Check sheet for the modelled part. Datum: model origin and axes. Units: mm. Face numbers are marked on the shaded views. Coordinates: 2 decimals unless noted, no trailing zeros. Loops run counter-clockwise (first coordinate to the right, second up) from the corner with the lowest first, then second, coordinate; pieces in that order, holes last. Notation, with made-up numbers: M 48.25,75.5 L 101.25,75.5 A30 ccw 101.25,113.5 Z; hole C 0.5,-35.75 d4. An arc over 180 degrees is marked long. Return JSON: item names as keys, results as strings.
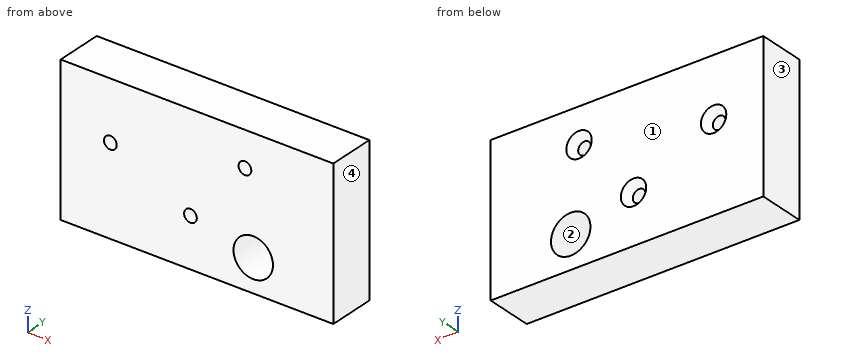
from build123d import *

# Parameters (mm, degrees)
F0_W           = 144.7047647089
F0_H           = 78.020889312
F0_R           = 10.4690892811
F0_R_2         = 14.6326120323
F1_DEPTH       = 25
F2_D           = 6.7564
F2_CSINK_D     = 13.4874
F2_CSINK_ANGLE = 82
F3_DEPTH       = 25


with BuildPart() as f1:
    # F0 (on Front) → F1 (new body)
    with BuildSketch(Plane.XZ):
        with Locations((-52.569960244, -12.6112531871)):
            Rectangle(F0_W, F0_H)
        with Locations((-22.7131489664, -34.2154763639)):
            Circle(F0_R, mode=Mode.SUBTRACT)
        with Locations((-71.8028619885, -2.9601538554)):
            Circle(F0_R_2, mode=Mode.SUBTRACT)
    extrude(amount=F1_DEPTH)

    # F2 (through all)
    with Locations(Plane(origin=(0, 0, 0), x_dir=(1, 0, 0), z_dir=(0, 1, 0))):
        with Locations((-98.5457673669, 4.8187081702), (-56.0501925647, 25.5219973624), (-27.109246701, -7.7437334694)):
            CounterSinkHole(F2_D / 2, F2_CSINK_D / 2, counter_sink_angle=F2_CSINK_ANGLE)

    # F0 (on Front) → F3 (join)
    with BuildSketch(Plane.XZ):
        with Locations((-71.8028619885, -2.9601538554)):
            Circle(F0_R_2)
    extrude(amount=F3_DEPTH)


solid = f1.part
1) Go/stop test with flat-tipped pins: pin 1 Ø17 at (x, z) = (-22.71, -34.22) entering from +Y; pin 2 Ø8 at (x, z) = (-56.05, -25.52) entering from +Y. Record where each tip stops, or that it passes through.
Answers:
{"pin 1": "through", "pin 2": "y = -3.15"}
2) Draft check along X on the marked faces 1, 2, 3 and 4. Enter one of: +X half, -X half, draft (parallel to the pull), parting line (faces both ways), or undercut.
Answers:
{"face 1": "draft", "face 2": "undercut", "face 3": "-X half", "face 4": "+X half"}
3) Section check A-A on z = -39.5. Record the cut outline in (x, y), then the cut area to 3 significant figures.
Answers:
{"outline": "M -124.92,-25 L -31.75,-25 L -31.75,0 L -124.92,0 Z; M -13.68,-25 L 19.78,-25 L 19.78,0 L -13.68,0 Z", "area": "3,170 mm²"}
4) Section check B-B on y = -7. Record the cut outline in (x, z), then the cut area to 3 significant figures.
Answers:
{"outline": "M -124.92,-51.62 L 19.78,-51.62 L 19.78,26.4 L -124.92,26.4 Z; hole C -98.55,-4.82 d6.76; hole C -56.05,-25.52 d6.76; hole C -22.71,-34.22 d20.94; hole C -27.11,7.74 d6.76", "area": "10,800 mm²"}
5) Scan lines: line 1 along X through (y, z) = (-17.25, -33.5); line 2 along X through (y, z) = (-3.75, -28); line 3 along X through (y, z) = (-16.25, -34.5). Record each from-to range of solid material in increasing order. Write a range as [from, to].
Answers:
{"line 1": "[-124.92, -33.16], [-12.27, 19.78]", "line 2": "[-124.92, -58.5], [-53.6, -31.14], [-14.29, 19.78]", "line 3": "[-124.92, -33.18], [-12.25, 19.78]"}
